Autodesk Inventor part; units mm, degrees
ref_plane "YZ Plane" through (0, 0, 0) normal (1, 0, 0) x (0, 1, 0)
ref_plane "XZ Plane" through (0, 0, 0) normal (0, 1, 0) x (-1, 0, 0)
ref_plane "XY Plane" through (0, 0, 0) normal (0, 0, 1) x (1, 0, 0)
sketch "Sketch1" plane through (0, 0, 0) normal (0, 1, 0) x (-1, 0, 0)
  line L0 (20, 45) -> (-20, 45)
  line L1 (-20, 45) -> (-20, -45)
  line L2 (-20, -45) -> (20, -45)
  line L3 (20, -45) -> (20, 45)
  line L4 (20, 45) -> (-20, -45) construction
  line L5 (-20, 45) -> (20, -45) construction
  arc A0 (-20, -45) -> (20, -45) centre (0, -45) ccw
  line L6 (20, -45) -> (52, -45)
  line L7 (52, -45) -> (52, 45)
  line L8 (52, 45) -> (20, 45)
  line L9 (20, 45) -> (20, -45)
  point P0 (0, 0)
  dimension "d0" = 40
  dimension "d1" = 90
  dimension "d7" = 32
  dimension "d8" = 90
extrude "Extrusion1" add sketch "Sketch1" along normal blind 3.6
sketch "Sketch2" plane through (0, 3.6, 0) normal (0, 1, 0) x (1, 0, 0)
  arc A0 (20, 45) -> (-20, 45) centre (0, 45) ccw
  circle A1 centre (0, 45) radius 5.15
  point P0 (0, 0)
  dimension "d4" = 10.3
extrude "Extrusion2" cut sketch "Sketch2" against normal blind 3.6
fillet "Fillet1" radius 4 4 edges at (-20, 1.8, -45) (-52, 1.8, -45) (-52, 1.8, 45) (20, 1.8, 45)
sketch "Sketch3" plane through (0, 0, 0) normal (0, -1, 0) x (1, 0, 0)
  line L0 (-48, 45) -> (16, 45)
  line L1 (-45, 45) -> (-15, 45)
  line L2 (-15, 45) -> (-15, -30)
  line L3 (-15, -30) -> (-45, -30)
  line L4 (-45, -30) -> (-45, 45)
  line L5 (-52, -41) -> (-52, 41)
  circle A0 centre (-5, 20) radius 16.25
  line L6 (20, 41) -> (20, -45)
  point P0 (0, 0)
  dimension "d10" = 30
  dimension "d11" = 75
  dimension "d12" = 7
  dimension "d13" = 32.5
  dimension "d14" = 25
  dimension "d15" = 25
extrude "Extrusion3" cut sketch "Sketch3" against normal blind 10
fillet "Fillet2" radius 2 3 edges at (-15, 1.8, 45) (-15, 1.8, 32.8087) (-15, 1.8, 7.1913)
sketch "Sketch4" plane through (0, 0, 0) normal (0, -1, 0) x (1, 0, 0)
  circle A0 centre (-27.5, -40.5) radius 1.625
  circle A1 centre (15.5, 40.5) radius 1.625
  circle A2 centre (15.5, -19.5) radius 1.625
  line L0 (20, 41) -> (20, -45)
  line L1 (-13, 45) -> (16, 45)
  line L2 (-23.6643, -45) -> (-48, -45)
  line L3 (-52, -41) -> (-52, 41)
  point P0 (0, 0)
  dimension "d19" = 3.25
  dimension "d20" = 3.25
  dimension "d21" = 3.25
  dimension "d22" = 4.5
  dimension "d23" = 4.5
  dimension "d24" = 4.5
  dimension "d25" = 60
  dimension "d26" = 4.5
  dimension "d27" = 24.5
extrude "Extrusion4" cut sketch "Sketch4" against normal blind 10
sketch "Sketch5" plane through (0, 3.6, 0) normal (0, 1, 0) x (1, 0, 0)
  circle A0 centre (-48, -40) radius 1.575
  line L0 (-52, 41) -> (-52, -41)
  line L1 (-13, -45) -> (16, -45)
  point P0 (0, 0)
  dimension "d30" = 3.15
  dimension "d31" = 4
  dimension "d32" = 5
extrude "Extrusion5" cut sketch "Sketch5" against normal blind 10
properties part number "p1"
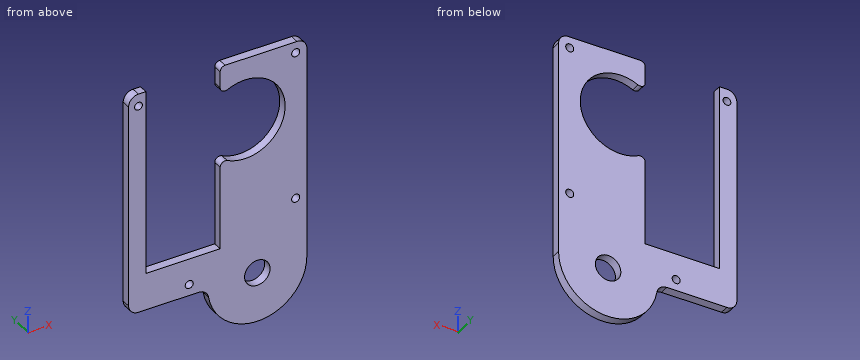
Could you check a few things on this model? Use its own coordinates, in mm. Round coordinates to 2 decimals unless told otherwise and drop trailing zeros. Order: outer loops, then holes, each group sorted by start corner. A loop starts at its lowest first (then second) coordinate and runs counter-clockwise, first axis right, second up.
(1) Please list where these lines run through material, in increasing order: line 1 along Z through (x, y) = (-48, 2.5) (3 decimals); line 2 along X through (y, z) = (2.05, -24); line 3 along Z through (x, y) = (15.5, 2.2) (3 decimals).
Response values:
line 1: z = -45 to 38.425, 41.575 to 45
line 2: x = -52 to -45, -15 to 20
line 3: z = -57.639 to -21.125, -17.875 to 38.875, 42.125 to 45
(2) I'm going to push a flat-ended pin straight in: pin 1 (1.1 mm diameter, centred on x = -34, y = 1.5, fed in from +Z). Where does the tip first touch, or does it pass through?
Response values:
pin 1: stops at z = -30
(3) Imagine slicing it at A-A (z = -19.5). Write out the boundary of the cut face in (x, y) (3 decimals), plus the area to 4 significant figures.
Response values:
outline: (-52, 0) - (-45, 0) - (-45, 3.6) - (-52, 3.6) - close; (-15, 0) - (13.875, 0) - (13.875, 3.6) - (-15, 3.6) - close; (17.125, 0) - (20, 0) - (20, 3.6) - (17.125, 3.6) - close
area: 139.5 mm2
(4) Imagine slicing it at B-B (y = 1.25). Write out the boundary of the cut face in (x, z) (3 decimals), plus the area to 3 significant figures.
Response values:
outline: (-52, -41) arc R4 ccw to (-48, -45) - (-23.664, -45) arc R4 cw to (-19.72, -48.333) arc R20 ccw to (20, -45) - (20, 41) arc R4 ccw to (16, 45) - (-13, 45) arc R2 ccw to (-15, 43) - (-15, 36.403) arc R2 ccw to (-12.123, 34.606) arc R16.25 cw (long way) to (-12.123, 5.394) arc R2 ccw to (-15, 3.597) - (-15, -30) - (-45, -30) - (-45, 45) - (-48, 45) arc R4 ccw to (-52, 41) - close; hole circle Ø3.15 at (-48, 40); hole circle Ø3.25 at (-27.5, -40.5); hole circle Ø10.3 at (0, -45); hole circle Ø3.25 at (15.5, -19.5); hole circle Ø3.25 at (15.5, 40.5)
area: 4,010 mm2
(5) Imagine slicing it at D-D (x = -22). Write out the boundary of the cut face in (y, z), plus the area to 3 significant figures.
Response values:
outline: (0, -45.36) - (3.6, -45.36) - (3.6, -30) - (0, -30) - close
area: 55.3 mm2
(6) Imagine slicing it at C-C (x = -39). Write out the boundary of the cut face in (y, z), plus the area to 3 significant figures.
Response values:
outline: (0, -45) - (3.6, -45) - (3.6, -30) - (0, -30) - close
area: 54.0 mm2
